Geometry check sheet. Reference: the model listing, model coordinates, mm. A direction names the side the tool comes from. Coordinates: 2 decimals unless noted, no trailing zeros. Write each loop counter-clockwise with the first axis right and the second up, starting at its lowest first coordinate (ties: lowest second). Pieces come first, ordered by that corner, then holes.
from build123d import *

# Parameters (mm, degrees)
F1_DEPTH  = 25.4
F3_DEPTH  = 25.4
F5_DEPTH  = 101.6
F7_DEPTH  = 127
F8_DEPTH  = 25.4
F10_DEPTH = 25.4


with BuildPart() as f1:
    # F0 (on Front) → F1 (new body)
    with BuildSketch(Plane.XZ):
        Polygon((25.4, 38.1), (0, 38.1), (0, 0), (69.502056, 0.486028), (69.502056, 12.7), (25.4, 12.7), align=None)
    extrude(amount=F1_DEPTH)

    # F2 (on face) → F3 (cut)
    with BuildSketch(Plane.XY.offset(12.7)):
        with BuildLine():
            ThreePointArc((56.802056, 0), (65.782312, -3.719744), (69.502056, -12.7))
            Line((69.502056, -12.7), (69.502056, 0))
            Line((69.502056, 0), (56.802056, 0))
        make_face()
        with BuildLine():
            Line((56.802056, -25.4), (69.502056, -25.4))
            Line((69.502056, -25.4), (69.502056, -12.7))
            ThreePointArc((69.502056, -12.7), (65.782312, -21.680256), (56.802056, -25.4))
        make_face()
    extrude(amount=-F3_DEPTH, mode=Mode.SUBTRACT)

    # F4 (on face) → F5 (cut)
    with BuildSketch(Plane.XZ.offset(25.4)):
        with BuildLine():
            ThreePointArc((6.357221, 27.282854), (12.548588, 20.631922), (19.05, 26.980117))
            ThreePointArc((19.05, 26.980117), (12.851412, 33.328312), (6.357221, 27.282854))
        make_face()
    extrude(amount=-F5_DEPTH, mode=Mode.SUBTRACT)

    # F6 (on face) → F7 (cut)
    with BuildSketch(Plane.XZ.offset(25.4)):
        with BuildLine():
            ThreePointArc((12.7, 38.1), (21.680256, 34.380256), (25.4, 25.4))
            Line((25.4, 25.4), (25.4, 38.1))
            Line((25.4, 38.1), (12.7, 38.1))
        make_face()
        with BuildLine():
            ThreePointArc((0, 25.4), (3.719744, 34.380256), (12.7, 38.1))
            Line((12.7, 38.1), (0, 38.1))
            Line((0, 38.1), (0, 25.4))
        make_face()
    extrude(amount=F7_DEPTH, mode=Mode.SUBTRACT)

    # F6 (on face) → F8 (cut)
    with BuildSketch(Plane.XZ.offset(25.4)):
        with BuildLine():
            ThreePointArc((0, 25.4), (3.719744, 34.380256), (12.7, 38.1))
            Line((12.7, 38.1), (0, 38.1))
            Line((0, 38.1), (0, 25.4))
        make_face()
        with BuildLine():
            ThreePointArc((12.7, 38.1), (21.680256, 34.380256), (25.4, 25.4))
            Line((25.4, 25.4), (25.4, 38.1))
            Line((25.4, 38.1), (12.7, 38.1))
        make_face()
    extrude(amount=-F8_DEPTH, mode=Mode.SUBTRACT)

    # F9 (on Top) → F10 (cut)
    with BuildSketch(Plane.XY):
        with BuildLine():
            ThreePointArc((63.5, -12.7), (61.640128, -8.209872), (57.15, -6.35))
            ThreePointArc((57.15, -6.35), (50.8, -12.7), (57.15, -19.05))
            ThreePointArc((57.15, -19.05), (61.640128, -17.190128), (63.5, -12.7))
        make_face()
        with BuildLine():
            ThreePointArc((38.1, -6.35), (42.590128, -8.209872), (44.45, -12.7))
            ThreePointArc((44.45, -12.7), (42.590128, -17.190128), (38.1, -19.05))
            Line((38.1, -19.05), (57.15, -19.05))
            ThreePointArc((57.15, -19.05), (50.8, -12.7), (57.15, -6.35))
            Line((57.15, -6.35), (38.1, -6.35))
        make_face()
        with BuildLine():
            ThreePointArc((38.1, -19.05), (42.590128, -17.190128), (44.45, -12.7))
            ThreePointArc((44.45, -12.7), (42.590128, -8.209872), (38.1, -6.35))
            ThreePointArc((38.1, -6.35), (31.75, -12.7), (38.1, -19.05))
        make_face()
    extrude(amount=F10_DEPTH, mode=Mode.SUBTRACT)


solid = f1.part
1. Thickness scan on line 1 along Y through (x, z) = (44, 8); line 2 along Z through (x, y) = (30.5, -18.5); line 3 along Z through (x, y) = (39, -2.75). Record the ranges inside material, lowest first.
Computed values:
line 1: y = -25.4 to -19.05, -6.35 to 0
line 2: z = 0.21 to 12.7
line 3: z = 0.27 to 12.7
2. Access from +Z, -Z, +X, -X, +Y, -Y to the whole of each face (thin tool, end or side, straight path). Record for faces 4 (the flat face through (0, -13, 13)), 5 (the cylindrical face through (31.75, -12.56, 6.37)).
Computed values:
face 4: +Z, -Z, -X, +Y, -Y
face 5: +Z, -Z
3. Sectioned sample at B-B, the plane z = 12. Record the boundary of the cut face in (x, y).
Computed values:
outline: (0, -25.4) - (56.8, -25.4) arc R12.7 ccw to (56.8, 0) - (0, 0) - close; hole (38.1, -19.05) - (57.15, -19.05) arc R6.35 ccw to (57.15, -6.35) - (38.1, -6.35) arc R6.35 ccw to start
4. Gauge pin test, flat ends, axial feed: pin 1 Ø1 at (y, z) = (-12.5, 18.5) entering from +X; pin 2 Ø5 at (y, z) = (-14, 28.5) entering from -X; pin 3 Ø2 at (x, y) = (21, -11.5) entering from -Z. Record the tip position at first contact, or that the pin passes through.
Computed values:
pin 1: stops at x = 25.4
pin 2: stops at x = 0.01
pin 3: stops at z = 0.14
5. Sectioned sample at C-C, the plane x = 41. Record the boundary of the cut face in (y, z).
Computed values:
outline: (-25.4, 0.29) - (-19.05, 0.29) - (-19.05, 12.7) - (-25.4, 12.7) - close; (-6.35, 0.29) - (0, 0.29) - (0, 12.7) - (-6.35, 12.7) - close
6. Sectioned sample at D-D, the plane z = 24.5. Record the boundary of the cut face in (x, y), and give its area (3 significant figures).
Computed values:
outline: (0, -25.4) - (6.85, -25.4) - (6.85, 0) - (0, 0) - close; (18.55, -25.4) - (25.4, -25.4) - (25.4, 0) - (18.55, 0) - close
area: 348 mm2
7. Sectioned sample at A-A, the plane y = -9. Record the boundary of the cut face in (x, z).
Computed values:
outline: (0, 0) - (32.94, 0.23) - (32.94, 12.7) - (25.4, 12.7) - (25.4, 25.4) arc R12.7 ccw to (0, 25.4) - close; (62.31, 0.44) - (68.95, 0.48) - (68.95, 12.7) - (62.31, 12.7) - close; hole (6.36, 27.28) arc R6.35 ccw (long way) to (19.05, 26.98) arc R6.35 ccw to start
8. Draft check along X on faces 1 (the flat face through (47, -19.05, 6)), 2 (the flat face through (25.4, -13, 19)), 3 (the flat face through (48, -21, 12.7)). Enter one of: released by +X, released by -X, zero draft, split by the parting line, or undercut.
Computed values:
face 1: undercut
face 2: released by +X
face 3: zero draft
